Could you check a few things on this drawing? It's one solid part, dimensions in mm from its lowest x, y, z. A direction names the side the tool comes from. Give positions to 0.01 mm unless a question says otherwise; leave off trailing zeros. Loops run counter-clockwise (first coordinate to the right, second up) from the corner with the lowest first, then second, coordinate; pieces in that order, holes last. Notation, with made-up numbers: (35.5, 56.25) - (80.5, 56.25) arc R24 ccw to (80.5, 81.25) - close; hole circle Ø2 at (64.5, -8). An arc over 180 degrees is marked (long way). Use a Markdown table: item, result.
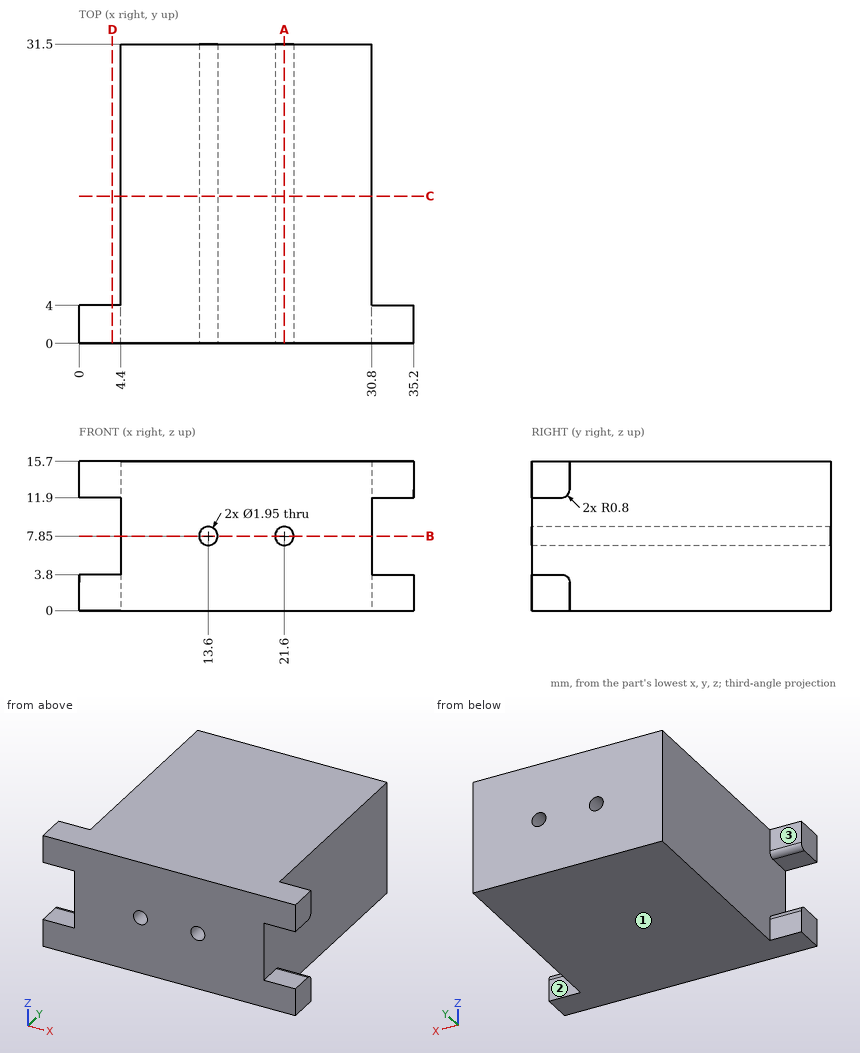
(1) If I drill on line 1 (X direction, y = 14, z = 7.85) (3 decimals); line 2 (X direction, y = 21, z = 2.25); line 3 (Y direction, x = 32, z = 13.75), over which ranges is the centre line in solid material (lowest first)?
A:
| item | result |
|---|---|
| line 1 | 4.4 to 12.625, 14.575 to 20.625, 22.575 to 30.8 |
| line 2 | 4.4 to 30.8 |
| line 3 | 0 to 4 |
(2) Will these pins go through, and if not, where does the flat tip stop? pin 1 (6 mm diameter, centred on y = 25, z = 12, fed in from -X); pin 2 (3 mm diameter, centred on y = 26, z = 5.5, fed in from +X); pin 3 (1.5 mm diameter, centred on x = 33.5, z = 2, fed in from +Y).
A:
| item | result |
|---|---|
| pin 1 | x = 4.4 |
| pin 2 | x = 30.8 |
| pin 3 | y = 4 |
(3) Suppose I cut it at C-C on y = 15.5. Write out the boundary of the cut face in (x, z) (3 decimals), plus the area to 3 significant figures.
A:
| item | result |
|---|---|
| outline | (4.4, 0) - (30.8, 0) - (30.8, 15.7) - (4.4, 15.7) - close; hole circle Ø1.95 at (13.6, 7.85); hole circle Ø1.95 at (21.6, 7.85) |
| area | 409 mm2 |
(4) Suppose I cut it at A-A on x = 21.6. Write out the boundary of the cut face in (y, z) (3 decimals).
A:
| item | result |
|---|---|
| outline | (0, 0) - (31.5, 0) - (31.5, 6.875) - (0, 6.875) - close; (0, 8.825) - (31.5, 8.825) - (31.5, 15.7) - (0, 15.7) - close |
(5) Suppose I cut it at D-D on x = 3.5. Write out the boundary of the cut face in (y, z).
A:
| item | result |
|---|---|
| outline | (0, 0) - (4, 0) - (4, 3) arc R0.8 ccw to (3.2, 3.8) - (0, 3.8) - close; (0, 11.9) - (3.2, 11.9) arc R0.8 ccw to (4, 12.7) - (4, 15.7) - (0, 15.7) - close |
(6) On a 3-axis mill with a long thin cutter (end or side, diameter ignored), from which of +Z, -Z, +X, -X, +Y, -Y can I reach the whole of each face in a straight line? I mean the marked faces 1, 2 and 3. Say none if no direction works.
A:
| item | result |
|---|---|
| face 1 | -Z, +X, -X, +Y, -Y |
| face 2 | +Z, -Z, +X, +Y |
| face 3 | +Z, -Z, -X, +Y |
(7) Suppose I cut it at B-B on z = 7.85. Write out the boundary of the cut face in (x, y) (3 decimals).
A:
| item | result |
|---|---|
| outline | (4.4, 0) - (12.625, 0) - (12.625, 31.5) - (4.4, 31.5) - close; (14.575, 0) - (20.625, 0) - (20.625, 31.5) - (14.575, 31.5) - close; (22.575, 0) - (30.8, 0) - (30.8, 31.5) - (22.575, 31.5) - close |
